from build123d import *

# Parameters (mm, degrees)
SKETCH1_R           = 3.3019999999999836
BOSS_EXTRUDE1_DEPTH = 1.5875
SKETCH2_R           = 12.7
CUT_EXTRUDE2_DEPTH  = 146.57558110485613
CUT_EXTRUDE3_DEPTH  = 400.917308055041
CUT_EXTRUDE4_DEPTH  = 400.91690405439095
FILLET1_R           = 1.5875


with BuildPart() as part:
    # Sketch1 → Boss-Extrude1 (new body)
    with BuildSketch(Plane(origin=(4.715e-14, 220.81273991226263, -315.3532743689599), x_dir=(-1, 7e-17, -1e-16), z_dir=(0, 0.5735764363510497, -0.8191520442889892))):
        with BuildLine():
            Line((-352.9368830837315, 115.82645369700992), (-375.29590907686907, 107.8750150529707))
            ThreePointArc((-375.29590907686907, 107.8750150529707), (-383.0064063960404, 91.65378726062865), (-366.7851786036984, 83.94328994145738))
            Line((-366.7851786036984, 83.94328994145738), (-352.9368830837315, 88.86809624497586))
            Line((-352.9368830837315, 88.86809624497586), (-352.9368830837315, 115.82645369700992))
        make_face()
        with Locations(Location((-375.5277422986924, 94.31339053349453, 0), (0, 0, 90))):
            Circle(SKETCH1_R, mode=Mode.SUBTRACT)
    extrude(amount=BOSS_EXTRUDE1_DEPTH)

    # Sketch2 → Cut-Extrude2 (cut, through all)
    with BuildSketch(Plane(origin=(364.35174229869244, 343.62540364794484, -135.39966553044988), x_dir=(-0.9960075449626111, 0.027318171664055604, 0.08498639817338811), z_dir=(-0.0892690897094424, -0.3047987291070713, -0.9482240053685426))):
        with Locations((-0.03783689084002617, -0.5075300251178305)):
            Circle(SKETCH2_R)
    extrude(amount=CUT_EXTRUDE2_DEPTH, mode=Mode.SUBTRACT)

    # Sketch3 → Cut-Extrude3 (cut, through all)
    with BuildSketch(Plane(origin=(4.734e-14, 221.72329250496995, -316.65367823926863), x_dir=(-1, 7e-17, -1e-16), z_dir=(0, 0.5735764363510497, -0.8191520442889892))):
        with BuildLine():
            Line((-361.4453353005722, 85.84227411038414), (-360.53395932333007, 86.16638260092915))
            Line((-360.53395932333007, 86.16638260092915), (-363.80419645721065, 111.96176050593412))
            add(Edge.make_bspline(
                [(-363.80419645721065, 111.96176050593412), (-368.8920523914014, 98.57905697453593), (-361.4453353005722, 85.84227411038414)],
                knots=[0.8633594194263924, 0.8633594194263924, 0.8633594194263924, 2.2053014206357777, 2.2053014206357777, 2.2053014206357777], degree=2, weights=[1, 0.7832183186966504, 1]))
        make_face()
    extrude(amount=-CUT_EXTRUDE3_DEPTH, mode=Mode.SUBTRACT)

    # Sketch5 → Cut-Extrude4 (cut, through all)
    with BuildSketch(Plane(origin=(4.715e-14, 220.81273991226263, -315.3532743689599), x_dir=(1, -7e-17, 1e-16), z_dir=(0, -0.5735764363510497, 0.8191520442889892))):
        with BuildLine():
            Line((364.81964209388303, 111.600642196092), (363.80419645721065, 111.96176050593412))
            Line((363.80419645721065, 111.96176050593412), (365.40184998669423, 99.04304749276544))
            add(Edge.make_bspline(
                [(365.40184998669423, 99.04304749276544), (366.3557730480568, 105.71124194209018), (364.81964209388303, 111.600642196092)],
                knots=[4.662458191197461, 4.662458191197461, 4.662458191197461, 5.280973611848554, 5.280973611848554, 5.280973611848554], degree=2, weights=[1, 0.9525597493758428, 1]))
        make_face()
    extrude(amount=-CUT_EXTRUDE4_DEPTH, mode=Mode.SUBTRACT)

    # Fillet1
    fillet1_edges = [part.edges().sort_by_distance(p)[0] for p in [
        (361.44533530057225, 291.5858905325532, -266.76637063161013),
        (364.8196420938831, 312.685910407509, -251.99197765879123),
    ]]
    fillet(fillet1_edges, radius=FILLET1_R)


solid = part.part
Can you work these out from the model? Positions are in its coordinate system, mm. Round coordinates to 2 decimals unless told otherwise and drop trailing zeros. Order: outer loops, then holes, each group sorted by start corner. A loop starts at its lowest first (then second) coordinate and runs counter-clockwise, first axis right, second up. Notation, with made-up numbers: (80, 29) - (86, 29) arc R18 ccw to (86, 55) - close; hole circle Ø6 at (-15.5, 60). An arc over 180 degrees is marked (long way). Answer in a Markdown table with one row per item.
(1) If we mould it in two halves opening along X, with no side actions, what happens to faces 1 (the face through (373.09, 300.41, -259.62)), 2 (the face through (371.33, 310.78, -253.31)), 3 (the face through (365.42, 302.41, -259.18)), 4 (the face through (372.304, 297.932, -262.309))? For each: released by +X, released by -X, zero draft, split by the parting line, or undercut.
From the geometry:
| item | result |
|---|---|
| face 1 | zero draft |
| face 2 | released by +X |
| face 3 | released by -X |
| face 4 | undercut |
(2) Suppose I cut it at C-C, the plane x = 370.75. Please give me the cut outline in (y, z), plus the area to 3 significant figures.
From the geometry:
| item | result |
|---|---|
| outline | (288.98, -267.62) - (289.89, -268.92) - (311.41, -253.85) - (310.5, -252.55) - close |
| area | 41.7 mm2 |
(3) Please list where these lines run through material, in increasing order: L1, parallel to Y at x = 372, z = -259; L2, parallel to Y at x = 376.75, z = -257.75; L3, parallel to Z at x = 379.5, y = 298.5. Write a range as from..to.
From the geometry:
| item | result |
|---|---|
| L1 | y = 301.29..304.06 |
| L2 | y = 303.08..305.85 |
| L3 | z = -262.89..-260.96 |
(4) For P1, Ø2, axis at y = 293, z = -267, coming from the +X side; P2, Ø8, axis at x = 373, z = -260.5, coming from the -Y side; P3, Ø5, axis at y = 301, z = -263, coming from the +X side; P4, Ø4, axis at y = 295.5, z = -266.5, coming from the +X side, each with a flat end and sliding along its axis, tell me the tip position at first contact or that it passes through.
From the geometry:
| item | result |
|---|---|
| P1 | stops at x = 380.85 |
| P2 | stops at y = 293.44 |
| P3 | stops at x = 383.74 |
| P4 | stops at x = 382.66 |
(5) Suppose I cut it at A-A, the plane x = 377. Please give me the cut outline in (y, z).
From the geometry:
| item | result |
|---|---|
| outline | (290.19, -266.77) - (291.1, -268.08) - (296.56, -264.25) - (295.65, -262.95) - close; (300.49, -259.56) - (301.4, -260.86) - (309.47, -255.21) - (308.56, -253.91) - close |
(6) Suppose I cut it at B-B, the plane x = 374.25. Please give me the cut outline in (y, z).
From the geometry:
| item | result |
|---|---|
| outline | (289.31, -267.39) - (290.22, -268.69) - (296.49, -264.3) - (295.58, -263) - close; (300.56, -259.51) - (301.47, -260.81) - (310.39, -254.57) - (309.48, -253.27) - close |
